Build history of the part. All positions in model axes, mm. Face numbers are marked on the shaded views. A direction names the side the tool comes from. Give positions to 0.01 mm unless a question says otherwise; leave off trailing zeros. Loops run counter-clockwise (first coordinate to the right, second up) from the corner with the lowest first, then second, coordinate; pieces in that order, holes last. Notation, with made-up numbers: M 6,17.25 L 63,17.25 A26 ccw 63,32.25 Z; hole C 9.25,34.5 d8. An arc over 180 degrees is marked long. Answer as a JSON object with one key per item and string values. Group by question number.
1. Slice it at D-D (x = 23). List the corners of the cut face in (y, z).
2. 3-axis set-ups, long thin cutter, end or side, ignore diameter. For the marked faces 1, 2 and 3: which of +Z, -Z, +X, -X, +Y, -Y reach the whole face in a straight line?
3. Mould opens along X. For the marked faces 4, 5 and 6 say: released by +X, released by -X, zero draft, split by the parting line, or undercut.
4. Drop flat-ended pins along their axis: pin 1 Ø8.5 at (x, y) = (2, -5) entering from +Z; pin 2 Ø3 at (x, z) = (-11, -17.5) entering from +Y; pin 3 Ø2 at (y, z) = (0.5, -21.5) entering from -X; pin 4 Ø2 at (x, y) = (-14.5, -5.5) entering from +Z. Give the stop position or say it passes through.
5. Slice it at A-A (x = 0). List the corners of the cut face in (y, z), then the cut area to 3 significant figures.
6. Slice it at C-C (z = -14.25). List the corners of the cut face in (x, y), then the cut area to 3 significant figures.
7. Drill centre lines: line 1 along Y through (x, z) = (0, -13.5); line 2 along Y through (x, z) = (-18, -5); line 3 along Y through (x, z) = (-18, -15.25). Where is each one in solid material? Low to high. Write a range as [from, to].
8. Slice it at B-B (y = 0). List the corners of the cut face in (x, z).
from build123d import *

# Parameters (mm, degrees)
SKETCH_R        = 14
SKETCH_R_2      = 2.75
PAD_DEPTH       = 17
SKETCH001_R     = 9
SKETCH001_R_2   = 2.75
PAD001_DEPTH    = 3
SKETCH002_R     = 3
SKETCH002_R_2   = 2.75
PAD002_DEPTH    = 2
CHAMFER_SIZE    = 0.5
CHAMFER001_SIZE = 1
SKETCH003_W     = 15
SKETCH003_H     = 5
POCKET_DEPTH    = 22.001
FILLET_R        = 1
PAD003_DEPTH    = 10


with BuildPart() as part:
    # Sketch → Pad (new body)
    with BuildSketch(Plane.XY):
        with BuildLine():
            ThreePointArc((-14.073185, 9.536533), (-23.781107, 6.605863), (-16.975525, -0.911891))
            ThreePointArc((-16.975525, -0.911891), (-0.931565, -16.974457), (16.773787, -2.764066))
            Line((16.773787, -2.764066), (26.176697, -0.883484))
            ThreePointArc((26.176697, -0.883484), (30.883484, 6.176697), (23.823303, 10.883484))
            Line((23.823303, 10.883484), (14.420394, 9.002902))
            ThreePointArc((14.420394, 9.002902), (0.318322, 16.997019), (-14.073185, 9.536533))
        make_face()
        Circle(SKETCH_R, mode=Mode.SUBTRACT)
        with Locations((25, 5)):
            Circle(SKETCH_R_2, mode=Mode.SUBTRACT)
        with Locations((-18, 5)):
            Circle(SKETCH_R_2, mode=Mode.SUBTRACT)
    extrude(amount=-PAD_DEPTH)

    # Sketch001 → Pad001 (join)
    with BuildSketch(Plane.XY.offset(-17)):
        with BuildLine():
            ThreePointArc((-14.073185, 9.536533), (-23.781107, 6.605863), (-16.975525, -0.911891))
            ThreePointArc((-16.975525, -0.911891), (-0.931565, -16.974457), (16.773787, -2.764066))
            Line((16.773787, -2.764066), (26.176697, -0.883484))
            ThreePointArc((26.176697, -0.883484), (30.883484, 6.176697), (23.823303, 10.883484))
            Line((23.823303, 10.883484), (14.420394, 9.002902))
            ThreePointArc((14.420394, 9.002902), (0.318322, 16.997019), (-14.073185, 9.536533))
        make_face()
        Circle(SKETCH001_R, mode=Mode.SUBTRACT)
        with Locations((25, 5)):
            Circle(SKETCH001_R_2, mode=Mode.SUBTRACT)
        with Locations((-18, 5)):
            Circle(SKETCH001_R_2, mode=Mode.SUBTRACT)
    extrude(amount=-PAD001_DEPTH)

    # Sketch002 → Pad002 (join)
    with BuildSketch(Plane.XY.offset(-20)):
        with BuildLine():
            ThreePointArc((-14.073185, 9.536533), (-23.781107, 6.605863), (-16.975525, -0.911891))
            ThreePointArc((-16.975525, -0.911891), (-0.931565, -16.974457), (16.773787, -2.764066))
            Line((16.773787, -2.764066), (26.176697, -0.883484))
            ThreePointArc((26.176697, -0.883484), (30.883484, 6.176697), (23.823303, 10.883484))
            Line((23.823303, 10.883484), (14.420394, 9.002902))
            ThreePointArc((14.420394, 9.002902), (0.318322, 16.997019), (-14.073185, 9.536533))
        make_face()
        Circle(SKETCH002_R, mode=Mode.SUBTRACT)
        with Locations((25, 5)):
            Circle(SKETCH002_R_2, mode=Mode.SUBTRACT)
        with Locations((-18, 5)):
            Circle(SKETCH002_R_2, mode=Mode.SUBTRACT)
    extrude(amount=-PAD002_DEPTH)

    # Chamfer
    chamfer_edges = [part.edges().sort_by_distance(p)[0] for p in [
        (-9, 0, -17),
    ]]
    chamfer(chamfer_edges, length=CHAMFER_SIZE)

    # Chamfer001
    chamfer001_edges = [part.edges().sort_by_distance(p)[0] for p in [
        (-3, 0, -20),
    ]]
    chamfer(chamfer001_edges, length=CHAMFER001_SIZE)

    # Sketch003 (on Face6 of Chamfer001) → Pocket (cut, through all)
    with BuildSketch(Plane(origin=(0, 0, -22), x_dir=(1, 0, 0), z_dir=(0, 0, -1))):
        Rectangle(SKETCH003_W, SKETCH003_H)
    extrude(amount=-POCKET_DEPTH, mode=Mode.SUBTRACT)

    # Fillet
    fillet_edges = [part.edges().sort_by_distance(p)[0] for p in [
        (-7.5, -2.5, -21),
        (7.5, -2.5, -21),
        (7.5, 2.5, -21),
        (-7.5, 2.5, -21),
    ]]
    fillet(fillet_edges, radius=FILLET_R)

    # Sketch004 (on Face15 of Fillet) → Pad003 (join)
    with BuildSketch(Plane(origin=(0, 0, -22), x_dir=(1, 0, 0), z_dir=(0, 0, -1))):
        with BuildLine():
            ThreePointArc((-17.738007, -13.175152), (-19.042066, -14.479211), (-17.738007, -15.78327))
            Line((-17.738007, -15.78327), (-5.033958, -15.78327))
            ThreePointArc((-5.033958, -15.78327), (-3.729899, -14.479211), (-5.033958, -13.175152))
            Line((-17.738007, -13.175152), (-5.033958, -13.175152))
        make_face()
    extrude(amount=-PAD003_DEPTH)


solid = part.part
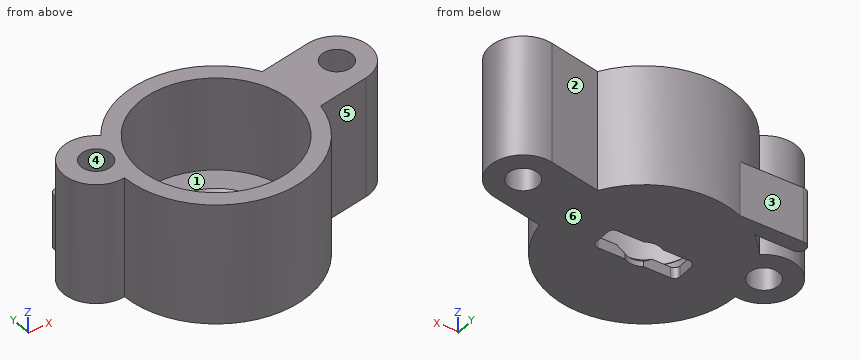
Established:
{
 "1": {"outline": "M -1.52,-22 L 3.11,-22 L 3.11,0 L -1.52,0 Z; M 6.89,-22 L 10.72,-22 L 10.72,0 L 6.89,0 Z"},
 "2": {"face 1": "+Z", "face 2": "+Z, -Z, +Y", "face 3": "+Z, -Z, -X, +Y"},
 "3": {"face 4": "undercut", "face 5": "released by +X", "face 6": "zero draft"},
 "4": {"pin 1": "stops at z = -17", "pin 2": "stops at y = 15.78", "pin 3": "stops at x = -22.87", "pin 4": "stops at z = 0"},
 "5": {"outline": "M -17,-22 L -3,-22 L -3,-21 L -4,-20 L -9,-20 L -9,-17.5 L -9.5,-17 L -14,-17 L -14,0 L -17,0 Z; M 3,-22 L 17,-22 L 17,0 L 14,0 L 14,-17 L 9.5,-17 L 9,-17.5 L 9,-20 L 4,-20 L 3,-21 Z", "area": "205 mm^2"},
 "6": {"outline": "M -17.74,13.18 L -10.74,13.18 A17 ccw -14.07,9.54 A6 ccw long -16.98,-0.91 A17 ccw 16.77,-2.76 L 26.18,-0.88 A6 ccw 23.82,10.88 L 14.42,9 A17 ccw -6.32,15.78 L -17.74,15.78 A1.3 ccw Z; hole C -18,5 d5.5; hole C 0,0 d28; hole C 25,5 d5.5", "area": "513 mm^2"},
 "7": {"line 1": "y = [-17, -14], [14, 17]", "line 2": "y = [-1, 2.25], [7.75, 11]", "line 3": "y = [-1, 2.25], [7.75, 11], [13.2, 15.76]"},
 "8": {"outline": "M -21.32,-22 L -7.5,-22 L -7.5,-20 L -9,-20 L -9,-17.5 L -9.5,-17 L -14,-17 L -14,0 L -21.32,0 Z; M 7.5,-22 L 28.32,-22 L 28.32,0 L 14,0 L 14,-17 L 9.5,-17 L 9,-17.5 L 9,-20 L 7.5,-20 Z"}
}
